Verification items for this drawing (mm, ordinates from the low corner). Coordinates: 2 decimals unless noted, no trailing zeros. Order: outer loops, then holes, each group sorted by start corner. A loop starts at its lowest first (then second) coordinate and runs counter-clockwise, first axis right, second up. Notation, with made-up numbers: (-27, -16.5) -> (5, -16.5) arc R20 cw to (5, 22.5) -> close; hole circle Ø11 at (13.25, 68). An arc over 180 degrees is marked (long way). Write each question's results on one line, items separated by ' | '. Start each with the question number.
(1) Draft check along Z on the marked faces 1, 2 and 3. Enter one of: +Z half, -Z half, draft (parallel to the pull), parting line (faces both ways), or undercut.
(2) Thickness scan on probe 1 along Y at (x, z) = (12.5, 2.75); probe 2 along Z at (x, y) = (20.5, 7.5); probe 3 along X at (y, z) = (11.75, 2.5). Record the ranges inside material, lowest first. Write a range as [from, to].
(3) Cross-section at A-A on y = 12.5. Enter the section's corners in (x, z).
(4) Cross-section at C-C on z = 2.75. Enter the section's corners in (x, y).
(5) Go/stop test with flat-tipped pins: pin 1 (1 mm diameter, centred on x = 5.5, y = 16, fed in from -Z); pin 2 (1 mm diameter, centred on y = 16, z = 4, fed in from +X); pin 3 (1 mm diameter, centred on y = 12.5, z = 4.5, fed in from -X). Record where each tip stops, or that it passes through.
(6) Cross-section at D-D on x = 2.75. Enter the section's corners in (y, z).
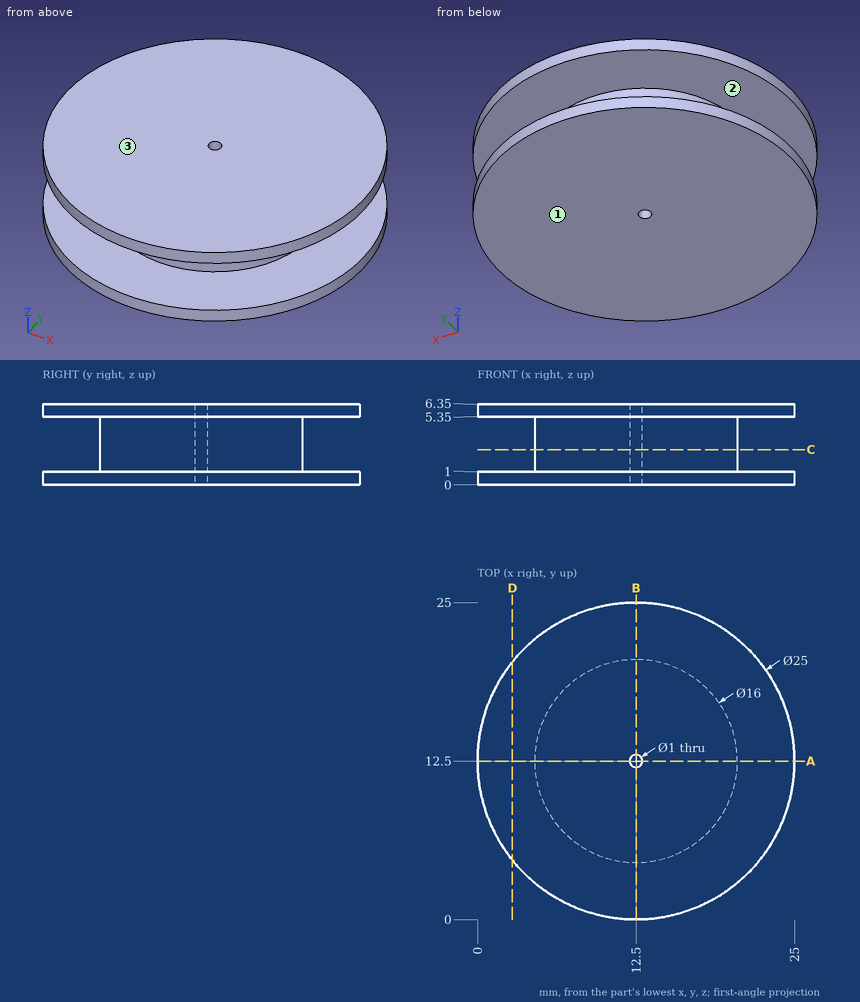
Results are:
1) face 1: -Z half | face 2: undercut | face 3: +Z half
2) probe 1: y = [4.5, 12], [13, 20.5] | probe 2: z = [0, 1], [5.35, 6.35] | probe 3: x = [4.54, 20.46]
3) outline: (0, 0) -> (12, 0) -> (12, 6.35) -> (0, 6.35) -> (0, 5.35) -> (4.5, 5.35) -> (4.5, 1) -> (0, 1) -> close; (13, 0) -> (25, 0) -> (25, 1) -> (20.5, 1) -> (20.5, 5.35) -> (25, 5.35) -> (25, 6.35) -> (13, 6.35) -> close
4) outline: circle Ø16 at (12.5, 12.5); hole circle Ø1 at (12.5, 12.5)
5) pin 1: stops at z = 0 | pin 2: stops at x = 19.92 | pin 3: stops at x = 4.5
6) outline: (4.68, 0) -> (20.32, 0) -> (20.32, 1) -> (4.68, 1) -> close; (4.68, 5.35) -> (20.32, 5.35) -> (20.32, 6.35) -> (4.68, 6.35) -> close
